The listing builds one solid part. Answer for the finished solid, in the listing's coordinates (mm). Give positions to 0.01 mm unless a question says otherwise; leave off trailing zeros. Loops run counter-clockwise (first coordinate to the right, second up) from the corner with the lowest first, then second, coordinate; pieces in that order, holes last.
Item 1: Consider line 1 along Y through (x, z) = (0, 0.45); line 2 along X through (y, z) = (47.5, 0.55); line 3 along X through (y, z) = (-14.5, 0.6). Determine where each line is inside the solid, lowest interval first.
Item 2: The mould has two halves that part along Y. Classify faces 1 (the face through (24.257, -43.076, 0.493)), 2 (the face through (24.59, 42.62, 0.49)), 3 (the face through (4.84, -42.41, 0.49)): pulls with the +Y half, pulls with the -Y half, needs draft (parallel to the pull), parting line crosses it, or undercut.
Item 3: Section D-D, the plane x = 16.5 is taken. Give the vertices of the cut face in (y, z).
Item 4: Section A-A, the plane x = 0 is taken. Give the vertices of the cut face in (y, z), and give its area (3 significant figures).
Item 5: Section C-C, the plane z = 0.5 is taken. Give the vertices of the cut face in (x, y) (3 decimals).
Item 6: Section B-B, the plane y = 0 is taken. Give the vertices of the cut face in (x, z), and give its area (3 significant figures).
from build123d import *

# Parameters (mm, degrees)
SKETCH1_R      = 20
SKETCH1_R_2    = 9
EXTRUDE1_DEPTH = 1


with BuildPart() as part:
    # Sketch1 → Extrude1 (new body)
    with BuildSketch(Plane.XY):
        with BuildLine():
            Line((-12.514750297, 59.145), (-36.333146024, 26.55))
            ThreePointArc((-36.333146024, 26.55), (-45, 0), (-36.333146024, -26.55))
            Line((-36.333146024, -26.55), (-12.514750297, -59.145))
            ThreePointArc((-12.514750297, -59.145), (0, -65.5), (12.514750297, -59.145))
            Line((12.514750297, -59.145), (36.333146024, -26.55))
            ThreePointArc((36.333146024, -26.55), (45, 0), (36.333146024, 26.55))
            Line((36.333146024, 26.55), (12.514750297, 59.145))
            ThreePointArc((12.514750297, 59.145), (0, 65.5), (-12.514750297, 59.145))
        make_face()
        Circle(SKETCH1_R, mode=Mode.SUBTRACT)
        with Locations((0, -50)):
            Circle(SKETCH1_R_2, mode=Mode.SUBTRACT)
        with Locations((0, 50)):
            Circle(SKETCH1_R_2, mode=Mode.SUBTRACT)
    extrude(amount=EXTRUDE1_DEPTH)


solid = part.part
Worked answers:
1. line 1: y = -65.5 to -59, -41 to -20, 20 to 41, 59 to 65.5
1. line 2: x = -21.02 to -8.65, 8.65 to 21.02
1. line 3: x = -42.6 to -13.77, 13.77 to 42.6
2. face 1: pulls with the -Y half
2. face 2: pulls with the +Y half
2. face 3: undercut
3. outline: (-53.69, 0) - (-11.3, 0) - (-11.3, 1) - (-53.69, 1) - close; (11.3, 0) - (53.69, 0) - (53.69, 1) - (11.3, 1) - close
4. outline: (-65.5, 0) - (-59, 0) - (-59, 1) - (-65.5, 1) - close; (-41, 0) - (-20, 0) - (-20, 1) - (-41, 1) - close; (20, 0) - (41, 0) - (41, 1) - (20, 1) - close; (59, 0) - (65.5, 0) - (65.5, 1) - (59, 1) - close
4. area: 55.0 mm2
5. outline: (-36.333, -26.55) - (-12.515, -59.145) arc R15.5 ccw to (12.515, -59.145) - (36.333, -26.55) arc R45 ccw to (36.333, 26.55) - (12.515, 59.145) arc R15.5 ccw to (-12.515, 59.145) - (-36.333, 26.55) arc R45 ccw to start; hole circle Ø40 at (0, 0); hole circle Ø18 at (0, -50); hole circle Ø18 at (0, 50)
6. outline: (-45, 0) - (-20, 0) - (-20, 1) - (-45, 1) - close; (20, 0) - (45, 0) - (45, 1) - (20, 1) - close
6. area: 50.0 mm2
